The model under review builds one solid part; all positions refer to its coordinate system, in mm. Round coordinates to 2 decimals unless told otherwise and drop trailing zeros. Loops run counter-clockwise (first coordinate to the right, second up) from the corner with the lowest first, then second, coordinate; pieces in that order, holes last. Notation, with made-up numbers: (-15.5, 64) -> (4.5, 64) arc R33 ccw to (4.5, 102) -> close; hole circle Ø11 at (61, 38). An arc over 180 degrees is marked (long way). Use a Markdown table: item, result. Add a question column.
1) Mouldability with a two-part tool opening along Z and no side actions: class faces 1 (the cylindrical face through (20.765, -4.93, -39.923)), 2 (the flat face through (9, -10, -19)), 3 (the flat face through (15, -5, 11)) as released by +Z, released by -Z, zero draft, split by the parting line, or undercut.
2) Consider section B-B on y = -8.75. State how many separate pieces and enclosed holes the cut face has, plus the area to 3 significant figures.
3) Insertion check: pin 1 (5 mm diameter, centred on y = -3, z = -15, fed in from -X); pin 2 (4.5 mm diameter, centred on x = 9.5, y = -5, fed in from -Z); pin 3 (4.5 mm diameter, centred on y = -7.5, z = -9, fed in from +X). Each pin has a flat end and moves straight along its axis. Give the tip position at first contact, or say it passes through.
4) Consider section A-A on x = 7.5. Give the boundary of the cut face in (y, z), plus the area to 3 significant figures.
5) Consider section C-C on x = -5. Give the boundary of the cut face in (y, z), plus the area to 3 significant figures.
6) Wall thickness on probe 1 along Z at (x, y) = (-0.5, -3.5); probe 2 along Z at (x, y) = (12, -1.75); probe 3 along X at (y, z) = (-0.75, 34): over which ranges is each line inside the solid? List them lowest first.
from build123d import *

# Parameters (mm, degrees)
F0_R     = 45
F0_R_2   = 3.5
F1_DEPTH = 10


with BuildPart() as f1:
    # F0 (on Front) → F1 (new body)
    with BuildSketch(Plane.XZ):
        Circle(F0_R)
        with Locations((-26.870058, -26.870058)):
            Circle(F0_R_2, mode=Mode.SUBTRACT)
        with Locations((-14.54197, -35.107422)):
            Circle(F0_R_2, mode=Mode.SUBTRACT)
        with Locations((-35.107422, -14.54197)):
            Circle(F0_R_2, mode=Mode.SUBTRACT)
        with Locations((0, -38)):
            Circle(F0_R_2, mode=Mode.SUBTRACT)
        with Locations((14.54197, -35.107422)):
            Circle(F0_R_2, mode=Mode.SUBTRACT)
        with Locations((26.870058, -26.870058)):
            Circle(F0_R_2, mode=Mode.SUBTRACT)
        with Locations((35.107422, -14.54197)):
            Circle(F0_R_2, mode=Mode.SUBTRACT)
        with Locations((-38, 0)):
            Circle(F0_R_2, mode=Mode.SUBTRACT)
        with Locations((-35.107422, 14.54197)):
            Circle(F0_R_2, mode=Mode.SUBTRACT)
        with Locations((-26.870058, 26.870058)):
            Circle(F0_R_2, mode=Mode.SUBTRACT)
        with Locations((-14.54197, 35.107422)):
            Circle(F0_R_2, mode=Mode.SUBTRACT)
        Polygon((15, 6.213203), (21.213203, 0), (15, -6.213203), (15, -15), (6.213203, -15), (0, -21.213203), (-6.213203, -15), (-15, -15), (-15, -6.213203), (-21.213203, 0), (-15, 6.213203), (-15, 15), (-6.213203, 15), (0, 21.213203), (6.213203, 15), (15, 15), align=None, mode=Mode.SUBTRACT)
        with Locations((38, 0)):
            Circle(F0_R_2, mode=Mode.SUBTRACT)
        with Locations((35.107422, 14.54197)):
            Circle(F0_R_2, mode=Mode.SUBTRACT)
        with Locations((0, 38)):
            Circle(F0_R_2, mode=Mode.SUBTRACT)
        with Locations((14.54197, 35.107422)):
            Circle(F0_R_2, mode=Mode.SUBTRACT)
        with Locations((26.870058, 26.870058)):
            Circle(F0_R_2, mode=Mode.SUBTRACT)
    extrude(amount=F1_DEPTH)


solid = f1.part
Result set:
| question | item | result |
|---|---|---|
| 1 | face 1 | split by the parting line |
| 1 | face 2 | zero draft |
| 1 | face 3 | undercut |
| 2 | separate pieces | 1 |
| 2 | enclosed holes | 17 |
| 2 | area | 4,690 mm2 |
| 3 | pin 1 | x = -43.23 |
| 3 | pin 2 | z = -44.41 |
| 3 | pin 3 | x = 44.49 |
| 4 | outline | (-10, -44.37) -> (0, -44.37) -> (0, -15) -> (-10, -15) -> close; (-10, 15) -> (0, 15) -> (0, 44.37) -> (-10, 44.37) -> close |
| 4 | area | 587 mm2 |
| 5 | outline | (-10, -44.72) -> (0, -44.72) -> (0, -16.21) -> (-10, -16.21) -> close; (-10, 16.21) -> (0, 16.21) -> (0, 44.72) -> (-10, 44.72) -> close |
| 5 | area | 570 mm2 |
| 6 | probe 1 | -45 to -41.46, -34.54 to -20.71, 20.71 to 34.54, 41.46 to 45 |
| 6 | probe 2 | -43.37 to -37.51, -32.7 to -15, 15 to 32.7, 37.51 to 43.37 |
| 6 | probe 3 | -29.48 to -17.86, -11.22 to 11.22, 17.86 to 29.48 |
